Check sheet for the modelled part. Datum: model origin and axes. Units: mm. Face numbers are marked on the shaded views. A direction names the side the tool comes from. Give positions to 0.01 mm unless a question says otherwise; leave off trailing zeros. Write each loop counter-clockwise with the first axis right and the second up, starting at its lowest first coordinate (ties: lowest second). Pieces come first, ordered by that corner, then holes. Notation, with made-up numbers: M 45.5,68 L 95.5,68 A12 cw 95.5,72 Z; hole C 40.5,13.25 d5. An arc over 180 degrees is marked long. Write item = value, one per line. Start each with the question number.
1) Sectioned sample at B-B, the plane x = 16.5. Count the separate pieces of the cut face and the enclosed holes in it, then the cut area to 3 significant figures.
2) Gauge pin test, flat ends, axial feed: pin 1 (2.5 mm diameter, centred on y = 4.76, z = 19.05, fed in from +X); pin 2 (3.5 mm diameter, centred on y = 4.76, z = 19.05, fed in from -X); pin 3 (8 mm diameter, centred on x = 0, z = -6.35, fed in from -Y); pin 4 (6 mm diameter, centred on x = 5.5, z = 3.18, fed in from +Y). Record the tip position at first contact, or that the pin passes through.
3) Sectioned sample at A-A, the plane z = -6.35. Record the cut outline in (x, y) (3 decimals).
4) Sectioned sample at C-C, the plane y = 8.25. Record the cut outline in (x, z) (3 decimals), then the cut area to 3 significant figures.
5) Scan lines: L1, parallel to Y at x = 13, z = 19 (3 decimals); L2, parallel to Y at x = 14.5, z = 19.05 (1 decimal); L3, parallel to Z at x = -17, y = 6 (3 decimals). Record each from-to range of solid material in increasing order.
6) Draft check along X on the marked faces 3, 4 and 5. Enter one of: pulls with the +X half, pulls with the -X half, needs draft (parallel to the pull), parting line crosses it, or undercut.
7) Set-up check for the marked faces 1 and 2: record each of +Z, -Z, +X, -X, +Y, -Y from which the full face is reachable in a straight line by a thin tool's end or side.
from build123d import *

# Parameters (mm, degrees)
SKETCH1_W                                            = 38.1
SKETCH1_H                                            = 57.15
BOSS_EXTRUDE1_DEPTH                                  = 9.525
CBORE_FOR_1_4_BINDING_HEAD_MACHINE_SCREW_D           = 6.7564
CBORE_FOR_1_4_BINDING_HEAD_MACHINE_SCREW_CBORE_D     = 14.2875
CBORE_FOR_1_4_BINDING_HEAD_MACHINE_SCREW_CBORE_DEPTH = 4.191
F_10_32_TAPPED_HOLE1_D                               = 4.0386
F_10_32_TAPPED_HOLE1_DEPTH                           = 12.7
F_10_32_TAPPED_HOLE1_CBORE_D                         = 4.826
F_10_32_TAPPED_HOLE1_CBORE_DEPTH                     = 9.652
F_10_32_TAPPED_HOLE1_TIP                             = 1.213317848
F_10_32_TAPPED_HOLE1_ON_FACE_2_D                     = 4.0386
F_10_32_TAPPED_HOLE1_ON_FACE_2_DEPTH                 = 12.7
F_10_32_TAPPED_HOLE1_ON_FACE_2_CBORE_D               = 4.826
F_10_32_TAPPED_HOLE1_ON_FACE_2_CBORE_DEPTH           = 9.652
F_10_32_TAPPED_HOLE1_ON_FACE_2_TIP                   = 1.213317848


with BuildPart() as part:
    # Sketch1 → Boss-Extrude1 (new body)
    with BuildSketch(Plane(origin=(0, 0, 0), x_dir=(1, 0, 0), z_dir=(0, 1, 0))):
        Rectangle(SKETCH1_W, SKETCH1_H)
    extrude(amount=BOSS_EXTRUDE1_DEPTH)

    # CBORE for 1/4 Binding Head Machine Screw1 (through all)
    with Locations(Plane(origin=(0, 0, 0), x_dir=(-1, 0, 0), z_dir=(0, -1, 0))):
        with Locations((0, 6.35), (5.499261314, -3.175), (-5.499261314, -3.175)):
            CounterBoreHole(CBORE_FOR_1_4_BINDING_HEAD_MACHINE_SCREW_D / 2, CBORE_FOR_1_4_BINDING_HEAD_MACHINE_SCREW_CBORE_D / 2, CBORE_FOR_1_4_BINDING_HEAD_MACHINE_SCREW_CBORE_DEPTH)

    # #10-32 Tapped Hole1
    with Locations(Plane(origin=(-19.05, 4.7625, -19.05), x_dir=(0, 0, -1), z_dir=(-1, 0, 0))):
        with Locations((0, 0), (-38.1, 0)):
            CounterBoreHole(F_10_32_TAPPED_HOLE1_D / 2, F_10_32_TAPPED_HOLE1_CBORE_D / 2, F_10_32_TAPPED_HOLE1_CBORE_DEPTH, depth=F_10_32_TAPPED_HOLE1_DEPTH)
            with Locations((0, 0, -(F_10_32_TAPPED_HOLE1_DEPTH + F_10_32_TAPPED_HOLE1_TIP / 2))):  # 118° drill point
                Cone(0, F_10_32_TAPPED_HOLE1_D / 2, F_10_32_TAPPED_HOLE1_TIP, mode=Mode.SUBTRACT)

    # #10-32 Tapped Hole1 on face 2
    with Locations(Plane(origin=(19.05, 4.7625, 19.05), x_dir=(0, 0, 1), z_dir=(1, 0, 0))):
        with Locations((0, 0), (-38.1, 0)):
            CounterBoreHole(F_10_32_TAPPED_HOLE1_ON_FACE_2_D / 2, F_10_32_TAPPED_HOLE1_ON_FACE_2_CBORE_D / 2, F_10_32_TAPPED_HOLE1_ON_FACE_2_CBORE_DEPTH, depth=F_10_32_TAPPED_HOLE1_ON_FACE_2_DEPTH)
            with Locations((0, 0, -(F_10_32_TAPPED_HOLE1_ON_FACE_2_DEPTH + F_10_32_TAPPED_HOLE1_ON_FACE_2_TIP / 2))):  # 118° drill point
                Cone(0, F_10_32_TAPPED_HOLE1_ON_FACE_2_D / 2, F_10_32_TAPPED_HOLE1_ON_FACE_2_TIP, mode=Mode.SUBTRACT)


solid = part.part
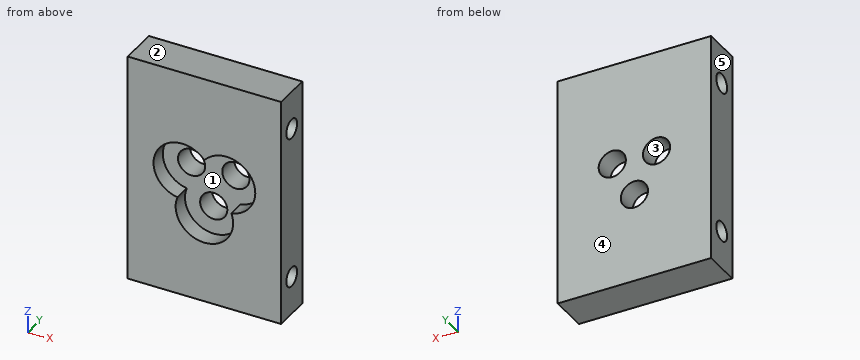
Data:
q1.separate_pieces = 1
q1.enclosed_holes = 2
q1.area = 508 mm2
q2.pin_1 = 5.89
q2.pin_2 = -6.19
q2.pin_3 = 4.19
q2.pin_4 = through
q3.outline = M -19.05,0 L -7.144,0 L -7.144,4.191 L -3.378,4.191 L -3.378,9.525 L -19.05,9.525 Z; M 3.378,4.191 L 7.144,4.191 L 7.144,0 L 19.05,0 L 19.05,9.525 L 3.378,9.525 Z
q4.outline = M -19.05,-28.575 L 19.05,-28.575 L 19.05,28.575 L -19.05,28.575 Z; hole C -5.499,3.175 d6.756; hole C 0,-6.35 d6.756; hole C 5.499,3.175 d6.756
q4.area = 2,070 mm2
q5.L1 = 0 to 2.35, 7.175 to 9.525
q5.L2 = 0 to 2.3, 7.2 to 9.5
q5.L3 = -28.575 to -21.122, -16.978 to 16.978, 21.122 to 28.575
q6.face_3 = undercut
q6.face_4 = needs draft
q6.face_5 = pulls with the -X half
q7.face_1 = -Y
q7.face_2 = +Z, +X, -X, +Y, -Y
